Work out the finished part from the listing and answer in its coordinate system (mm). Coordinates: 2 decimals unless noted, no trailing zeros. Write each loop counter-clockwise with the first axis right and the second up, starting at its lowest first coordinate (ties: lowest second). Pieces come first, ordered by that corner, then holes. Notation, with made-up numbers: (-22.5, 16) - (4.5, 16) arc R22 cw to (4.5, 49) - close; hole circle Ø6 at (30.25, 42.5). An arc over 180 degrees is marked (long way). Use a Markdown table: item, result. Add a question column.
(1) The part is cut by section A-A, the plane z = 58.5. State how many separate pieces and enclosed holes the cut face has, then the cut area to 3 significant figures.
(2) The part is cut by section B-B, the plane z = 130.5. Give the vertices of the cut face in (x, y), then the cut area to 3 significant figures.
(3) The part is cut by section D-D, the plane x = 0.5. Give the vertices of the cut face in (y, z), then the cut area to 3 significant figures.
(4) The part is cut by section C-C, the plane y = 3. Give the vertices of the cut face in (x, z), then the cut area to 3 significant figures.
(5) Given pin 1 Ø3 at (x, y) = (13, 21.5) entering from +Z (3 decimals); pin 2 Ø2.5 at (y, z) = (-15.5, 80.5) entering from -X; pin 3 Ø12 at (y, z) = (21, 116.5) entering from +X; pin 4 Ø5 at (x, z) = (-7.5, 82) entering from -Y, each flat-ended and moving along its own axis, determine where each tip first touches the part or whether it passes through.
(6) Find the intervals of material crossed by line 1 (Z direction, x = 15, y = 15); line 2 (Z direction, x = -19, y = -8); line 3 (Y direction, x = -22, z = 64), in increasing order. Write a range as from..to.
from build123d import *

# Parameters (mm, degrees)
F1_DEPTH = 20
F3_DEPTH = 50
F5_DEPTH = 90
F8_DEPTH = 1


with BuildPart() as f1:
    # F0 (on Top) → F1 (new body)
    with BuildSketch(Plane.XY):
        Polygon((-19.75, -17.7500005811), (-19.75, -19.75), (-13.75, -19.75), (19.75, 13.75), (19.75, 19.75), (17.7500005811, 19.75), (17.7500005811, 14.578426884), (-14.578426884, -17.7500005811), align=None)
    extrude(amount=F1_DEPTH)

    # F2 (on face) → F3 (join)
    with BuildSketch(Plane.XY.offset(20)):
        Polygon((-19.75, -19.75), (-13.75, -19.75), (19.75, 13.75), (19.75, 19.75), (11.25, 19.75), (11.25, 23.75), (7.75, 27.9211375741), (7.75, 24.8096899204), (9.25, 23.0220595315), (9.25, 19.75), (7.75, 19.75), (7.75, 17.7500005811), (14.3357871391, 11.164213442), (-11.164213442, -14.3357871391), (-17.7500005811, -7.75), (-19.75, -7.75), (-19.75, -9.25), (-23.0220595315, -9.25), (-24.8096899204, -7.75), (-27.9211375741, -7.75), (-23.75, -11.25), (-19.75, -11.25), align=None)
        Polygon((-17.7500005811, -17.7500005811), (-17.7500005811, -10.5784263029), (-12.5784265935, -15.7500002906), (-14.578426884, -17.7500005811), align=None, mode=Mode.SUBTRACT)
        Polygon((10.5784263029, 17.7500005811), (17.7500005811, 17.7500005811), (17.7500005811, 14.578426884), (15.7500002906, 12.5784265935), align=None, mode=Mode.SUBTRACT)
    extrude(amount=F3_DEPTH)

    # F4 (on face) → F5 (join)
    with BuildSketch(Plane.XY.offset(70)):
        Polygon((19.75, 13.75), (19.75, 19.75), (17.7500005811, 19.75), (17.7500005811, 14.578426884), (-14.578426884, -17.7500005811), (-19.75, -17.7500005811), (-19.75, -19.75), (-13.75, -19.75), align=None)
    extrude(amount=F5_DEPTH)

    # F7 (on mid) → F8 (join, symmetric)
    with BuildSketch(Plane.XY.offset(45)):
        Polygon((-23.0220595315, -9.25), (-19.75, -9.25), (-19.75, -7.75), (-24.8096899204, -7.75), align=None)
        Polygon((7.75, 19.75), (9.25, 19.75), (9.25, 23.0220595315), (7.75, 24.8096899204), align=None)
        Polygon((17.7500005811, 14.578426884), (17.7500005811, 17.7500005811), (10.5784263029, 17.7500005811), (15.7500002906, 12.5784265935), align=None)
        Polygon((-12.5784265935, -15.7500002906), (-17.7500005811, -10.5784263029), (-17.7500005811, -17.7500005811), (-14.578426884, -17.7500005811), align=None)
    extrude(amount=F8_DEPTH, both=True)


solid = f1.part
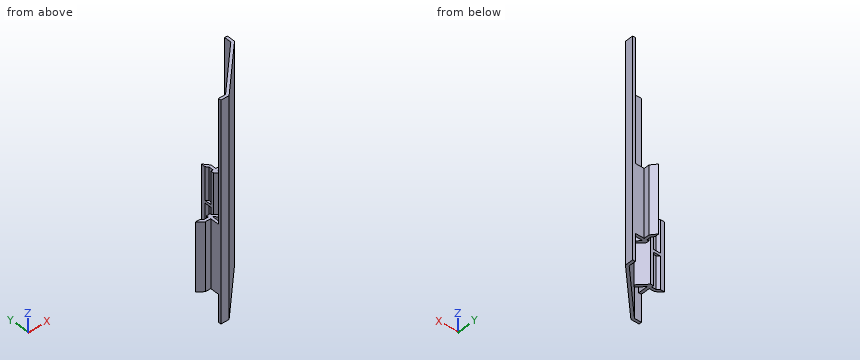
Model answer:
| question | item | result |
|---|---|---|
| 1 | separate pieces | 1 |
| 1 | enclosed holes | 2 |
| 1 | area | 219 mm^2 |
| 2 | outline | (-19.75, -19.75) - (-13.75, -19.75) - (19.75, 13.75) - (19.75, 19.75) - (17.75, 19.75) - (17.75, 14.58) - (-14.58, -17.75) - (-19.75, -17.75) - close |
| 2 | area | 115 mm^2 |
| 3 | outline | (-5.5, 0) - (-2.67, 0) - (-2.67, 160) - (-5.5, 160) - close |
| 3 | area | 453 mm^2 |
| 4 | outline | (6.17, 0) - (9, 0) - (9, 160) - (6.17, 160) - close |
| 4 | area | 453 mm^2 |
| 5 | pin 1 | through |
| 5 | pin 2 | x = -13.58 |
| 5 | pin 3 | x = 19.75 |
| 5 | pin 4 | y = -16 |
| 6 | line 1 | 44..46 |
| 6 | line 2 | 20..70 |
| 6 | line 3 | -11.25..-9.25 |
